Part model, mm, in its own coordinate system. Face numbers are marked on the shaded views. A direction names the side the tool comes from. Coordinates: 2 decimals unless noted, no trailing zeros. Loops run counter-clockwise (first coordinate to the right, second up) from the corner with the lowest first, then second, coordinate; pieces in that order, holes last. Notation, with made-up numbers: (-25, -14) -> (20, -14) arc R25 cw to (20, 20) -> close; hole circle Ø9 at (-14.5, 4). An arc over 180 degrees is marked (long way). One line per item, written item: value. Start each with the question number.
Autodesk Inventor part; units mm, degrees
ref_plane "YZ Plane" through (0, 0, 0) normal (1, 0, 0) x (0, 1, 0)
ref_plane "XZ Plane" through (0, 0, 0) normal (0, 1, 0) x (-1, 0, 0)
ref_plane "XY Plane" through (0, 0, 0) normal (0, 0, 1) x (1, 0, 0)
sketch "Sketch1" plane through (0, 0, 0) normal (0, 1, 0) x (-1, 0, 0)
  line L0 (0, 16.637) -> (17.0688, 16.637)
  line L1 (17.0688, 16.637) -> (17.0688, 14.9733)
  line L2 (39.8272, 14.9733) -> (39.8272, 16.637)
  line L3 (39.8272, 16.637) -> (56.896, 16.637)
  line L4 (56.896, 16.637) -> (56.896, 9.1604)
  line L5 (56.896, 9.1604) -> (56.896, 0)
  line L6 (56.896, 0) -> (0, 0)
  line L7 (0, 0) -> (0, 9.1604)
  line L8 (0, 9.1604) -> (13.556, 8.7368)
  line L9 (13.556, 8.7368) -> (13.556, 11.7983)
  line L10 (56.896, 9.1604) -> (43.34, 8.7368)
  line L11 (43.34, 8.7368) -> (43.34, 11.7983)
  line L12 (0, 9.1604) -> (0, 16.637)
  line L13 (17.0688, 16.637) -> (28.448, 16.637) construction
  line L14 (28.448, 16.637) -> (39.8272, 16.637) construction
  line L15 (28.448, 16.637) -> (28.448, 0) construction
  line L16 (17.0688, 14.9733) -> (28.448, 14.9733)
  line L17 (28.448, 14.9733) -> (39.8272, 14.9733)
  line L18 (13.556, 11.7983) -> (28.448, 11.7983)
  line L19 (28.448, 11.7983) -> (43.34, 11.7983)
  line L20 (37.6084, 28.448) -> (45.085, 28.448)
  line L21 (45.085, 28.448) -> (45.085, 11.3792)
  line L22 (45.085, 11.3792) -> (43.4213, 11.3792)
  line L23 (43.4213, 11.3792) -> (43.4213, 0)
  line L24 (43.4213, 0) -> (40.2463, 0)
  line L25 (37.6084, 28.448) -> (37.1848, 14.892)
  line L26 (37.6084, 28.448) -> (28.448, 28.448)
  line L27 (40.2463, 0) -> (28.448, 0)
  line L28 (28.448, 28.448) -> (28.448, 0) construction
  line L29 (37.1848, 14.892) -> (40.2463, 14.892)
  line L30 (40.2463, 14.892) -> (40.2463, 0)
  line L31 (13.556, 11.7983) -> (13.556, 0)
  line L32 (43.34, 11.7983) -> (43.34, 0)
  line L33 (40.2463, 14.892) -> (28.448, 14.892)
  line L34 (28.448, 14.892) -> (28.448, 0)
  line L35 (28.448, 28.448) -> (28.448, 14.892)
  dimension "d0" = 18.3208
  dimension "d1" = 33.274
  dimension "d2" = 17.0688
  dimension "d3" = 28.448
  dimension "d4" = 13.556
  dimension "d5" = 23.5966
  dimension "d6" = 3.175
  dimension "d7" = 1.79
  dimension "d8" = 28.448
  dimension "d9" = 17.0688
  dimension "d10" = 33.274
  dimension "d12" = 18.3208
  dimension "d13" = 23.5966
  dimension "d14" = 13.556
  dimension "d15" = 1.79
  dimension "d16" = 3.175
revolve "Revolve1" add sketch "Sketch1" angle 360 about axis through (-56.896, 0, 0) along (1, 0, 0) contours L0 L1 L16 L35 L34 L18 L9 L8 L12 | L8 L31 L6 L7 | L9 L18 L34 L6 L31 | L17 L25 L33 L35 | L17 L2 L3 L21 L22 L23 L10 L11 L19 L30 L29 L25 | L33 L29 L30 L19 L34 | L34 L19 L30 L6 | L30 L19 L11 L32 L6 | L32 L10 L23 L6 | L3 L4 L10 L23 L22 L21 | L23 L10 L5 L6
revolve "Revolve2" add sketch "Sketch1" angle 360 about axis through (-28.448, 0, 28.448) along (0, 0, -1) contours L25 L20 L21 L3 L2 L17 | L17 L2 L3 L21 L22 L23 L10 L11 L19 L30 L29 L25 | L33 L29 L30 L19 L34 | L34 L19 L30 L6 | L30 L19 L11 L32 L6 | L32 L10 L23 L6
revolve "Revolve3" cut sketch "Sketch1" angle 360 about axis through (-56.896, 0, 0) along (1, 0, 0) contours L8 L31 L6 L7 | L9 L18 L34 L6 L31 | L34 L19 L30 L6 | L30 L19 L11 L32 L6 | L32 L10 L23 L6 | L23 L10 L5 L6
revolve "Revolve4" cut sketch "Sketch1" angle 360 about axis through (-28.448, 0, 28.448) along (0, 0, -1) contours L35 L26 L25 L17 | L17 L25 L33 L35 | L33 L29 L30 L19 L34 | L34 L19 L30 L6
thread "Thread1"
thread "Thread2"
thread "Thread3"
equation "\"d0\" = MD"
equation "\"d1\" = H"
equation "\"d2\" = 0.6 * A"
equation "\"d3\" = A"
equation "\"d4\" = L2"
equation "\"d5\" = 0.9 * H - 2 * G"
equation "\"d6\" = G"
equation "\"d8\" = A"
equation "\"d9\" = 0.6 * A"
equation "\"d10\" = H"
equation "\"d12\" = MD"
equation "\"d13\" = 0.9 * H - 2 * G"
equation "\"d14\" = L2"
equation "\"d16\" = G"
equation "\"A\" = 28.448"
equation "\"L2\" = 13.55598"
equation "\"G\" = 3.175"
equation "\"H\" = 33.274"
equation "\"MD\" = 18.32077"
equation "\"Size_Designation\" = 0.5"
properties part number "ASME B16.11 Tee Threaded - Class 2000 1/2" material "Steel"
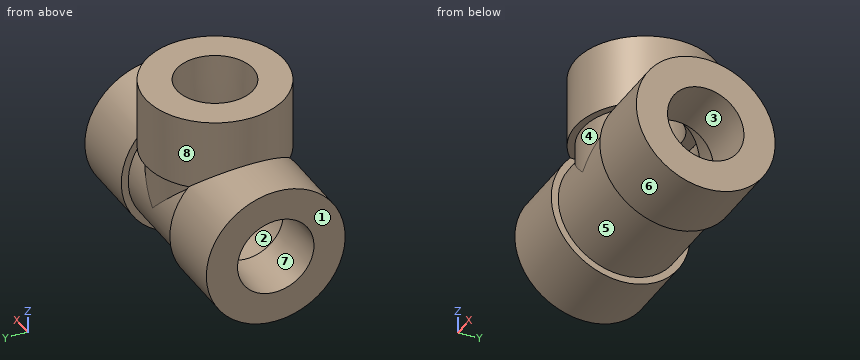
1) Slice it at A-A (y = -11). Give the cut face in (x, z), then the cut area to 3 significant figures.
2) Pull direction X, two halves, no side cores. Call the marked faces 1, 2 and 3: +X half, -X half, draft (parallel to the pull), parting line (faces both ways), or undercut.
3) Slice it at B-B (z = 20.5). Give the cut face in (x, y) (3 decimals).
4) Probe line 1 (Z direction, x = -27, y = 0); line 2 (Y direction, x = -12.5, z = -13.5); line 3 (X direction, y = -7.5, z = -7). List the from-to ranges inside material, lowest first. Write a range as from..to.
5) Tool access for the marked faces 4, 5, 6, 7 and 8: list every direction of +Z, -Z, +X, -X, +Y, -Y with a clear straight run to the whole face (end or side of a thin tool).
6) Slice it at D-D (y = 14). Give the cut face in (x, z).
7) Slice it at C-C (x = -52.5). Give the cut face in (y, z), then the cut area to 3 significant figures.
8) Pin check, flat tips, straight feed: pin 1 Ø12 at (y, z) = (5, 3) entering from +X; pin 2 Ø1 at (x, y) = (-50.5, 11.5) entering from +Z; pin 3 Ø7.5 at (x, y) = (-28.5, -14) entering from -Z (3 decimals); pin 4 Ø1.5 at (x, z) = (-18.5, 15) entering from -Y. Stop position of each tip, or through.
Check sheet entries:
1. outline: (-56.9, -12.48) -> (-39.83, -12.48) -> (-39.83, -10.16) -> (-17.07, -10.16) -> (-17.07, -12.48) -> (0, -12.48) -> (0, 12.48) -> (-15.97, 12.48) -> (-15.97, 28.45) -> (-40.93, 28.45) -> (-40.93, 12.48) -> (-56.9, 12.48) -> close; hole (-43.34, -4.27) -> (-13.56, -4.27) -> (-13.56, 4.27) -> (-24.18, 4.27) -> (-24.18, 14.89) -> (-32.71, 14.89) -> (-32.71, 4.27) -> (-43.34, 4.27) -> close; hole (-39.83, 10.16) -> (-38.61, 10.16) -> (-38.61, 11.38) -> (-39.83, 11.38) -> close; hole (-18.29, 10.16) -> (-17.07, 10.16) -> (-17.07, 11.38) -> (-18.29, 11.38) -> close
1. area: 1,420 mm^2
2. face 1: -X half
2. face 2: undercut
2. face 3: +X half
3. outline: circle Ø33.274 at (-28.448, 0); hole circle Ø17.824 at (-28.448, 0)
4. line 1: z = -14.97..-11.8
4. line 2: y = -9.72..9.72
4. line 3: x = -56.9..-43.34, -13.56..0
5. face 4: -Y
5. face 5: none
5. face 6: +X
5. face 7: -X
5. face 8: +Z
6. outline: (-56.9, -8.99) -> (-39.83, -8.99) -> (-39.83, -5.31) -> (-17.07, -5.31) -> (-17.07, -8.99) -> (0, -8.99) -> (0, 8.99) -> (-17.07, 8.99) -> (-17.07, 5.31) -> (-23.14, 5.31) -> (-23.14, 11.38) -> (-19.46, 11.38) -> (-19.46, 28.45) -> (-37.44, 28.45) -> (-37.44, 11.38) -> (-33.76, 11.38) -> (-33.76, 5.31) -> (-39.83, 5.31) -> (-39.83, 8.99) -> (-56.9, 8.99) -> close
7. outline: circle Ø33.27 at (0, 0); hole circle Ø18.05 at (0, 0)
7. area: 614 mm^2
8. pin 1: stops at x = 0
8. pin 2: stops at z = 12.48
8. pin 3: stops at z = -10.915
8. pin 4: stops at y = -13.86
